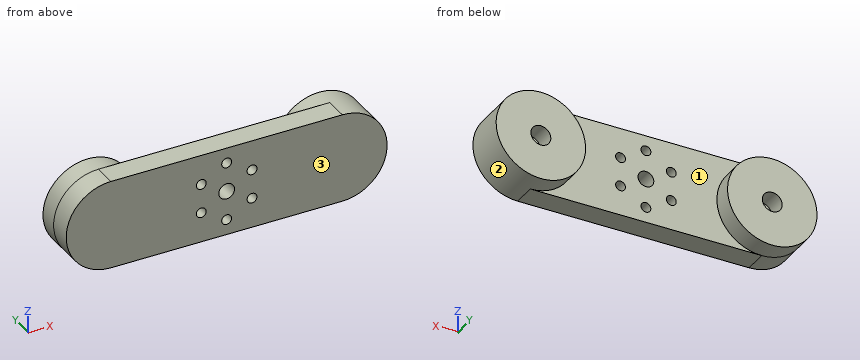
from build123d import *

# Parameters (mm, degrees)
SKETCH1_R            = 2.55
BOSS_EXTRUDE1_DEPTH  = 7.5
BOSS_EXTRUDE2_START  = 6.35
SKETCH1_3_R          = 2.55
SKETCH1_3_R_2        = 14.5
SKETCH1_3_R_3        = 3.225
BOSS_EXTRUDE2_DEPTH  = 6.35
M3_CLEARANCE_HOLE1_D = 3.2


with BuildPart() as part:
    # Sketch1 → Boss-Extrude1 (new body)
    with BuildSketch(Plane(origin=(0, 0, 0), x_dir=(1, 0, 0), z_dir=(0, 1, 0))):
        with BuildLine():
            Line((37.5, 14.5), (-37.5, 14.5))
            ThreePointArc((-37.5, 14.5), (-52, 0), (-37.5, -14.5))
            Line((-37.5, -14.5), (37.5, -14.5))
            ThreePointArc((37.5, -14.5), (52, 0), (37.5, 14.5))
        make_face()
        with Locations(Location((0, 0, 0), (0, 0, 270))):
            Circle(SKETCH1_R, mode=Mode.SUBTRACT)
    extrude(amount=-BOSS_EXTRUDE1_DEPTH)

    # Sketch1_3 → Boss-Extrude2 (add)
    # profile 1 of 3: a face of its own
    with BuildSketch(Plane(origin=(0, 0, 0), x_dir=(1, 0, 0), z_dir=(0, 1, 0)).offset(BOSS_EXTRUDE2_START)):
        with Locations(Location((0, 0, 0), (0, 0, 270))):
            Circle(SKETCH1_3_R)
    # profile 2 of 3: a face of its own
    with BuildSketch(Plane(origin=(0, 0, 0), x_dir=(1, 0, 0), z_dir=(0, 1, 0)).offset(BOSS_EXTRUDE2_START)):
        with Locations(Location((-37.5, 0, 0), (0, 0, 270))):
            Circle(SKETCH1_3_R_2)
        with Locations(Location((-37.5, 0, 0), (0, 0, 270))):
            Circle(SKETCH1_3_R_3, mode=Mode.SUBTRACT)
    # profile 3 of 3: a face of its own
    with BuildSketch(Plane(origin=(0, 0, 0), x_dir=(1, 0, 0), z_dir=(0, 1, 0)).offset(BOSS_EXTRUDE2_START)):
        with Locations(Location((37.5, 0, 0), (0, 0, 270))):
            Circle(SKETCH1_3_R_2)
        with Locations(Location((37.5, 0, 0), (0, 0, 270))):
            Circle(SKETCH1_3_R_3, mode=Mode.SUBTRACT)
    extrude(amount=-BOSS_EXTRUDE2_DEPTH)


with BuildPart() as boss_extrude2_kept_piece:
    # of the separate pieces the step leaves, the one the design keeps (boss_extrude2_pieces_kept)
    add(part.part.solids().sort_by_distance((-37.5, 0, 14.5))[0])

    # M3 Clearance Hole1 (through all)
    with Locations(Plane(origin=(-8.227241336, 0, -4.75), x_dir=(0, 0, 1), z_dir=(0, 1, 0))):
        with Locations((0, 0), (-4.75, 8.227241336), (0, 16.454482672), (9.5, 0), (9.5, 16.454482672), (14.25, 8.227241336)):
            Hole(M3_CLEARANCE_HOLE1_D / 2)


solid = boss_extrude2_kept_piece.part
Geometry check sheet. Reference: the model listing, model coordinates, mm. Face numbers are marked on the shaded views. Round coordinates to 2 decimals unless told otherwise and drop trailing zeros. Loops run counter-clockwise (first coordinate to the right, second up) from the corner with the lowest first, then second, coordinate; pieces in that order, holes last.
Item 1: Thickness scan on line 1 (Z direction, x = -7, y = -3.75); line 2 (X direction, y = -4.25, z = -4.75); line 3 (X direction, y = -4.5, z = 4.5). Record the ranges inside material, lowest first.
Item 2: Gauge pin test, flat ends, axial feed: pin 1 (8 mm diameter, centred on x = 0, z = 0, fed in from +Y); pin 2 (2 mm diameter, centred on x = 24.5, y = 0.5, fed in from -Z); pin 3 (6 mm diameter, centred on y = -1, z = 7.5, fed in from +X). Record the tip position at first contact, or that the pin passes through.
Item 3: Cross-section at C-C on z = -4.75. Record the boundary of the cut face in (x, y).
Item 4: Mould release check, pull along X, two halves, no side actions. Record for the marked faces 1, 2 and 3: pulls with the +X half, pulls with the -X half, needs draft (parallel to the pull), parting line crosses it, or undercut.
Item 5: Cross-section at A-A on z = 0. Record the boundary of the cut face in (x, y) (3 decimals).
Item 6: Cross-section at D-D on x = 26. Record the boundary of the cut face in (y, z).
Item 7: Cross-section at B-B on y = -2.5. Record the boundary of the cut face in (x, z).
Answer sheet:
1. line 1: z = -14.5 to -5.78, -3.72 to 3.72, 5.78 to 14.5
1. line 2: x = -51.2 to -9.83, -6.63 to 6.63, 9.83 to 51.2
1. line 3: x = -51.28 to -9.81, -6.65 to 6.65, 9.81 to 51.28
2. pin 1: stops at y = 0
2. pin 2: stops at z = -14.5
2. pin 3: stops at x = 51.28
3. outline: (-51.2, -7.5) - (-9.83, -7.5) - (-9.83, 0) - (-23.8, 0) - (-23.8, 6.35) - (-51.2, 6.35) - close; (-6.63, -7.5) - (6.63, -7.5) - (6.63, 0) - (-6.63, 0) - close; (9.83, -7.5) - (51.2, -7.5) - (51.2, 6.35) - (23.8, 6.35) - (23.8, 0) - (9.83, 0) - close
4. face 1: undercut
4. face 2: undercut
4. face 3: needs draft
5. outline: (-52, -7.5) - (-2.55, -7.5) - (-2.55, 0) - (-23, 0) - (-23, 6.35) - (-34.275, 6.35) - (-34.275, 0) - (-40.725, 0) - (-40.725, 6.35) - (-52, 6.35) - close; (2.55, -7.5) - (52, -7.5) - (52, 6.35) - (40.725, 6.35) - (40.725, 0) - (34.275, 0) - (34.275, 6.35) - (23, 6.35) - (23, 0) - (2.55, 0) - close
6. outline: (-7.5, -14.5) - (0, -14.5) - (0, -8.83) - (6.35, -8.83) - (6.35, 8.83) - (0, 8.83) - (0, 14.5) - (-7.5, 14.5) - close
7. outline: (-37.5, -14.5) - (37.5, -14.5) arc R14.5 ccw to (37.5, 14.5) - (-37.5, 14.5) arc R14.5 ccw to start; hole circle Ø3.2 at (-8.23, -4.75); hole circle Ø3.2 at (-8.23, 4.75); hole circle Ø5.1 at (0, 0); hole circle Ø3.2 at (0, -9.5); hole circle Ø3.2 at (0, 9.5); hole circle Ø3.2 at (8.23, -4.75); hole circle Ø3.2 at (8.23, 4.75)
